```python
from build123d import *

# Parameters (mm, degrees)
BOSS_EXTRUDE1_DEPTH = 0.44


with BuildPart() as part:
    # Sweep2: sweep along a path in Sketch1
    with BuildLine(Plane(origin=(0, 0, 0), x_dir=(1, 0, 0), z_dir=(0, 1, 0))) as sweep2_path:
        Line((7, 7), (10.80344393, 5.331523369))
        ThreePointArc((10.80344393, 5.331523369), (12, 3.5), (10.80344393, 1.668476631))
        Line((10.80344393, 1.668476631), (7, 0))
        Line((7, 0), (0, 0))
        Line((0, 0), (0, 7))
        Line((0, 7), (7, 7))
    # Sketch2 → Sweep2 (sweep)
    with BuildSketch(Plane(origin=(0, 0, 0), x_dir=(0, 0, -1), z_dir=(1, 0, 0))):
        with BuildLine():
            Line((0, 0), (0, 0.11))
            ThreePointArc((0, 0.11), (0.458946824, 0.771312392), (0.62, 1.56))
            Line((0.62, 1.56), (1.88, 1.56))
            Line((1.88, 1.56), (1.88, 1.12))
            Line((1.88, 1.12), (0.88, 1.12))
            Line((0.88, 1.12), (0.44, 0))
            Line((0.44, 0), (0, 0))
        make_face()
    sweep(path=sweep2_path.line, transition=Transition.RIGHT)

    # Sketch9 → Boss-Extrude1 (add)
    with BuildSketch(Plane(origin=(0, 1.56, 0), x_dir=(1, 0, 0), z_dir=(0, 1, 0))):
        with BuildLine():
            Line((6.605777013, 1.88), (10.048206636, 3.390108598))
            ThreePointArc((10.048206636, 3.390108598), (10.12, 3.5), (10.048206636, 3.609891402))
            Line((10.048206636, 3.609891402), (6.605777013, 5.12))
            Line((6.605777013, 5.12), (1.88, 5.12))
            Line((1.88, 5.12), (1.88, 1.88))
            Line((1.88, 1.88), (6.605777013, 1.88))
        make_face()
    extrude(amount=-BOSS_EXTRUDE1_DEPTH)


solid = part.part
```
Source: CAD feature listing. Evaluate the final solid. Frame: model axes, mm. A direction names the side the tool comes from. Give positions to 0.01 mm unless a question says otherwise; leave off trailing zeros. Loops run counter-clockwise (first coordinate to the right, second up) from the corner with the lowest first, then second, coordinate; pieces in that order, holes last. Notation, with made-up numbers: (18.25, -21.5) - (71.25, -21.5) arc R28 cw to (71.25, 2.5) - close; hole circle Ø4 at (11, 46.25). An arc over 180 degrees is marked (long way). Use CSV: the item, a comma, the result in double quotes.
1) Cut plane C-C (z = -3.5). Output: boundary loops of the cut face in (x, y).
Worked out:
outline,"(0, 0) - (0.44, 0) - (0.88, 1.12) - (11.12, 1.12) - (11.56, 0) - (12, 0) - (12, 0.11) arc R2 cw to (11.38, 1.56) - (0.62, 1.56) arc R2 cw to (0, 0.11) - close"
2) Cut plane B-B (x = 2.75). Output: boundary loops of the cut face in (y, z), and give its area (3 significant figures).
Worked out:
outline,"(0, -7) - (0.11, -7) arc R2 cw to (1.56, -6.38) - (1.56, -0.62) arc R2 cw to (0.11, 0) - (0, 0) - (0, -0.44) - (1.12, -0.88) - (1.12, -6.12) - (0, -6.56) - close"
area,"3.32 mm^2"
3) Cut plane D-D (y = 0.95). Output: boundary loops of the cut face in (x, z), and give its area (3 significant figures).
Worked out:
outline,"(0.53, -6.47) - (6.89, -6.47) - (10.59, -4.85) arc R1.47 ccw to (10.59, -2.15) - (6.89, -0.53) - (0.53, -0.53) - close; hole (0.81, -6.19) - (6.83, -6.19) - (10.48, -4.59) arc R1.19 ccw to (10.48, -2.41) - (6.83, -0.81) - (0.81, -0.81) - close"
area,"8.39 mm^2"
4) Set-up query: faces 5 (the flat face through (5, 1.56, -4)), 6 (the flat face through (8.65, 0.55, -1.44)). Return all of +Z, -Z, +X, -X, +Y, -Y with unobstructed straight access to the full face (end or side cutting, diameter ignored); none if empty.
Worked out:
face 5,"+Z, -Z, +X, -X, +Y"
face 6,"-Y"
5) Pin query (flat end, axial travel): P1, Ø1, axis at x = 6.5, z = -3, coming from the -Y side; P2, Ø4, axis at x = 10, z = -1.5, coming from the -Y side. Return the tip coordinate at first contact, or that it passes through.
Worked out:
P1,"stops at y = 1.12"
P2,"stops at y = 0"
6) Mould query, pull axis X, two halves, no side actions, for faces 1 (the cylindrical face through (0.463, 0.782, -3.549)), 2 (the conical face through (11.29, 0.69, -3.52)), 3 (the cylindrical face through (3.451, 0.782, -0.463)), 4 (the cylindrical face through (8.689, 0.782, -1.247)). Classes: +X half, -X half, draft (parallel to the pull), parting line (faces both ways), or undercut.
Worked out:
face 1,"-X half"
face 2,"undercut"
face 3,"draft"
face 4,"+X half"
7) Cut plane A-A (y = 0.4). Output: boundary loops of the cut face in (x, z).
Worked out:
outline,"(0.25, -6.75) - (6.95, -6.75) - (10.7, -5.1) arc R1.75 ccw to (10.7, -1.9) - (6.95, -0.25) - (0.25, -0.25) - close; hole (0.6, -6.4) - (6.87, -6.4) - (10.56, -4.78) arc R1.4 ccw to (10.56, -2.22) - (6.87, -0.6) - (0.6, -0.6) - close"
8) Line query: line 1 (Y direction, x = 3.25, z = -1.25); line 2 (Z direction, x = 10.5, y = 0.8); line 3 (X direction, y = 0.4, z = -2.5). Output: solid intervals per line, ascending.
Worked out:
line 1,"y = 1.12 to 1.56"
line 2,"z = -4.95 to -4.64, -2.36 to -2.05"
line 3,"x = 0.25 to 0.6, 10.98 to 11.44"
